from build123d import *

# Parameters (mm, degrees)
SKETCH1_R           = 6
BOSS_EXTRUDE1_DEPTH = 3
SKETCH2_R           = 6
CUT_EXTRUDE1_DEPTH  = 4


with BuildPart() as part:
    # Sketch1 → Boss-Extrude1 (new body)
    with BuildSketch(Plane(origin=(0, 0, 0), x_dir=(1, 0, 0), z_dir=(0, 1, 0))):
        with BuildLine():
            Line((-7.092556659, 19.326923077), (87.907443341, 19.326923077))
            ThreePointArc((87.907443341, 19.326923077), (97.907443341, 9.326923077), (87.907443341, -0.673076923))
            Line((87.907443341, -0.673076923), (-7.092556659, -0.673076923))
            ThreePointArc((-7.092556659, -0.673076923), (-17.092556659, 9.326923077), (-7.092556659, 19.326923077))
        make_face()
        with Locations((-7.092556659, 9.326923077)):
            Circle(SKETCH1_R, mode=Mode.SUBTRACT)
        with Locations((87.907443341, 9.326923077)):
            Circle(SKETCH1_R, mode=Mode.SUBTRACT)
    extrude(amount=BOSS_EXTRUDE1_DEPTH)

    # Sketch2 → Cut-Extrude1 (cut, through all)
    with BuildSketch(Plane(origin=(0, 3, 0), x_dir=(1, 0, 0), z_dir=(0, 1, 0))):
        with Locations((40.407443341, 9.326923077)):
            Circle(SKETCH2_R)
    extrude(amount=-CUT_EXTRUDE1_DEPTH, mode=Mode.SUBTRACT)


solid = part.part
Geometry check sheet. Reference: the model listing, model coordinates, mm. Give positions to 0.01 mm unless a question says otherwise; leave off trailing zeros. Loops run counter-clockwise (first coordinate to the right, second up) from the corner with the lowest first, then second, coordinate; pieces in that order, holes last. Notation, with made-up numbers: M 56.5,-29 L 90.5,-29 A25 cw 90.5,-4 Z; hole C -5.5,-17.75 d1. An arc over 180 degrees is marked long. Answer as a JSON object with one key per item and string values. Group by question number.
Item 1: Material ranges on L1, parallel to X at y = 2.35, z = -9.75; L2, parallel to X at y = 0.4, z = -13.25; L3, parallel to Z at x = -8, y = 1.55, recorded low to high.
Item 2: Sectioned sample at B-B on y = 1.9. Record the boundary of the cut face in (x, z).
Item 3: Sectioned sample at C-C on z = -13.75. Record the boundary of the cut face in (x, y), plus the area to 3 significant figures.
Item 4: Sectioned sample at A-A on z = -5.25. Record the boundary of the cut face in (x, y).
Item 5: Mould release check, pull along Z, two halves, no side actions. Record for faces 1 (the flat face through (41, 0, -3)), 2 (the cylindrical face through (-3.87, 1.48, -14.39)), 3 (the flat face through (41, 1, 0.673)): pulls with the +Z half, pulls with the -Z half, needs draft (parallel to the pull), parting line crosses it, or undercut.
Findings below:
{
 "1": {"L1": "-17.08 to -13.08, -1.11 to 34.42, 46.39 to 81.92, 93.89 to 97.9", "L2": "-16.29 to -11.63, -2.55 to 35.87, 44.95 to 83.37, 92.45 to 97.11", "L3": "-19.29 to -15.26, -3.4 to 0.63"},
 "2": {"outline": "M -7.09,-19.33 L 87.91,-19.33 A10 ccw 87.91,0.67 L -7.09,0.67 A10 ccw Z; hole C -7.09,-9.33 d12; hole C 40.41,-9.33 d12; hole C 87.91,-9.33 d12"},
 "3": {"outline": "M -16.06,0 L -11.15,0 L -11.15,3 L -16.06,3 Z; M -3.04,0 L 36.35,0 L 36.35,3 L -3.04,3 Z; M 44.46,0 L 83.85,0 L 83.85,3 L 44.46,3 Z; M 91.96,0 L 96.88,0 L 96.88,3 L 91.96,3 Z", "area": "266 mm2"},
 "4": {"outline": "M -16.22,0 L -11.49,0 L -11.49,3 L -16.22,3 Z; M -2.69,0 L 36.01,0 L 36.01,3 L -2.69,3 Z; M 44.81,0 L 83.51,0 L 83.51,3 L 44.81,3 Z; M 92.31,0 L 97.04,0 L 97.04,3 L 92.31,3 Z"},
 "5": {"face 1": "needs draft", "face 2": "undercut", "face 3": "pulls with the +Z half"}
}
